from build123d import *

# Parameters (mm, degrees)
BOSS_EXTRUDE1_DEPTH     = 70
CUT_EXTRUDE2_DEPTH      = 72.282887147
CUT_EXTRUDE2_DEPTH_BACK = 72.282887147
SKETCH2_R               = 2.5
FILLET1_SIZE            = 20
FILLET1_SIZE_2          = 15


with BuildPart() as part:
    # Sketch1 → Boss-Extrude1 (new body)
    with BuildSketch(Plane.XY):
        Polygon((6.5, 2.5), (12.5, 2.5), (12.5, -2.5), (-12.5, -2.5), (-12.5, 2.5), align=None)
    extrude(amount=BOSS_EXTRUDE1_DEPTH)

    # Sketch2 → Cut-Extrude2 (cut, two sides: drawn at the far end of the back side and taken through both)
    with BuildSketch(Plane(origin=(0, 2.5, 0), x_dir=(1, 0, 0), z_dir=(0, 1, 0)).offset(-CUT_EXTRUDE2_DEPTH_BACK)):
        with Locations(Location((-7.5, -5, 0), (0, 0, 270))):
            Circle(SKETCH2_R)
        with Locations(Location((-7.5, -20, 0), (0, 0, 270))):
            Circle(SKETCH2_R)
        with Locations(Location((-7.5, -35, 0), (0, 0, 270))):
            Circle(SKETCH2_R)
        with Locations(Location((-7.5, -50, 0), (0, 0, 270))):
            Circle(SKETCH2_R)
        with Locations(Location((-7.5, -65, 0), (0, 0, 270))):
            Circle(SKETCH2_R)
        with Locations(Location((2, -35, 0), (0, 0, 270))):
            Circle(SKETCH2_R)
    extrude(amount=CUT_EXTRUDE2_DEPTH + CUT_EXTRUDE2_DEPTH_BACK, mode=Mode.SUBTRACT)

    # Fillet1
    # an asymmetric fillet: 20, 15 mm, written as the material it takes off along each edge
    with BuildSketch(Plane(origin=(12.5, 52.5, 70), x_dir=(0, 0, -1), z_dir=(0, -1, 0))) as fillet1_piece_1:
        with BuildLine():
            Bezier((FILLET1_SIZE, 0), (0, 0), (0, -FILLET1_SIZE_2), weights=[1, 0.707106781, 1])
            Line((0, -FILLET1_SIZE_2), (0, 0))
            Line((0, 0), (FILLET1_SIZE, 0))
        make_face()
    extrude(amount=105, mode=Mode.SUBTRACT)
    with BuildSketch(Plane(origin=(12.5, 52.5, 0), x_dir=(0, 0, 1), z_dir=(0, -1, 0))) as fillet1_piece_2:
        with BuildLine():
            Bezier((FILLET1_SIZE, 0), (0, 0), (0, FILLET1_SIZE_2), weights=[1, 0.707106781, 1])
            Line((0, FILLET1_SIZE_2), (0, 0))
            Line((0, 0), (FILLET1_SIZE, 0))
        make_face()
    extrude(amount=105, mode=Mode.SUBTRACT)


solid = part.part
The listing builds one solid part. Answer for the finished solid, in the listing's coordinates (mm). Give positions to 0.01 mm unless a question says otherwise; leave off trailing zeros. Write each loop counter-clockwise with the first axis right and the second up, starting at its lowest first coordinate (ties: lowest second). Pieces come first, ordered by that corner, then holes. Notation, with made-up numbers: (-25.75, 89.25) -> (15.25, 89.25) arc R27 cw to (15.25, 115.25) -> close; hole circle Ø2 at (-6, 86.5). An arc over 180 degrees is marked (long way). Use a Markdown table: item, result.
(1) Find the intervals of material crossed by probe 1 along Z at (x, y) = (-7.5, 0.85); probe 2 along X at (y, z) = (-0.65, 35); probe 3 along X at (y, z) = (0.95, 50), in increasing order. Write a range as from..to.
Return value:
| item | result |
|---|---|
| probe 1 | 0..2.5, 7.5..17.5, 22.5..32.5, 37.5..47.5, 52.5..62.5, 67.5..70 |
| probe 2 | -12.5..-10, -5..-0.5, 4.5..12.5 |
| probe 3 | -12.5..-10, -5..12.5 |
(2) Section B-B, the plane z = 35 is taken. Determine the outline of the cut face in (x, y).
Return value:
| item | result |
|---|---|
| outline | (-12.5, -2.5) -> (-10, -2.5) -> (-10, 2.5) -> (-12.5, 2.5) -> close; (-5, -2.5) -> (-0.5, -2.5) -> (-0.5, 2.5) -> (-5, 2.5) -> close; (4.5, -2.5) -> (12.5, -2.5) -> (12.5, 2.5) -> (4.5, 2.5) -> close |
(3) Section A-A, the plane x = -9 is taken. Determine the outline of the cut face in (y, z).
Return value:
| item | result |
|---|---|
| outline | (-2.5, 0) -> (2.5, 0) -> (2.5, 3) -> (-2.5, 3) -> close; (-2.5, 7) -> (2.5, 7) -> (2.5, 18) -> (-2.5, 18) -> close; (-2.5, 22) -> (2.5, 22) -> (2.5, 33) -> (-2.5, 33) -> close; (-2.5, 37) -> (2.5, 37) -> (2.5, 48) -> (-2.5, 48) -> close; (-2.5, 52) -> (2.5, 52) -> (2.5, 63) -> (-2.5, 63) -> close; (-2.5, 67) -> (2.5, 67) -> (2.5, 70) -> (-2.5, 70) -> close |
(4) Determine the mould class of faces 1 (the flat face through (-7, 0, 0)), 2 (the cylindrical face through (1.04, -0.03, 37.31)), 3 (the flat face through (12.5, 0, 35)), 4 (the cylindrical face through (-8.46, -0.03, 37.31)) for opening direction Z: released by +Z, released by -Z, zero draft, split by the parting line, or undercut.
Return value:
| item | result |
|---|---|
| face 1 | released by -Z |
| face 2 | undercut |
| face 3 | zero draft |
| face 4 | undercut |
(5) Section C-C, the plane y = -1.35 is taken. Give the number of separate pieces and of enclosed holes in the cut face, then the cut area to 3 significant figures.
Return value:
| item | result |
|---|---|
| separate pieces | 1 |
| enclosed holes | 6 |
| area | 1,500 mm2 |
(6) Flat-ended cylindrical pins translate along their axes: P1, Ø3, axis at x = 10, y = -1, coming from the -Z side; P2, Ø6, axis at x = -7.5, z = 65, coming from the -Y side; P3, Ø3, axis at x = -7.5, z = 20, coming from the -Y side. Find the tip coordinate at first contact, or state that the pin passes through.
Return value:
| item | result |
|---|---|
| P1 | z = 6.4 |
| P2 | y = -2.5 |
| P3 | through |
